Here's how the part is built. I have some questions about the finished solid (model axes, mm). Round coordinates to 2 decimals unless told otherwise and drop trailing zeros. Write each loop counter-clockwise with the first axis right and the second up, starting at its lowest first coordinate (ties: lowest second). Pieces come first, ordered by that corner, then holes. Notation, with made-up numbers: M 87,52.25 L 95,52.25 A27 ccw 95,80.25 Z; hole C 54,1.5 d4. An arc over 180 degrees is marked long. Use a Markdown table: item, result. Add a question column.
```python
from build123d import *

# Parameters (mm, degrees)
F0_R        = 7.2334484139
F1_DEPTH    = 67.7
F2_R        = 15.3458789883
F3_DEPTH    = 21.4
F4_R        = 2
F5_S5_R     = 7.2334484139
F5_T6_DEPTH = 24
F6_R        = 5


# Not quite as in the source:
# - a fillet or chamfer that OpenCascade refuses, or shapes differently, is made with other operations: its cross-section is extruded or revolved along the edge and cut away or added


with BuildPart() as f1:
    # F0 (on Top) → F1 (new body)
    with BuildSketch(Plane.XY):
        Circle(F0_R)
    extrude(amount=F1_DEPTH)

    # F2 (on Top) → F3 (join)
    with BuildSketch(Plane.XY):
        Circle(F2_R)
    extrude(amount=F3_DEPTH)

    # F4
    f4_edges = [f1.edges().sort_by_distance(p)[0] for p in [
        (-7.233448, 0, 67.7),
    ]]
    fillet(f4_edges, radius=F4_R)

    # F5: chamfer of 10 on 1 edges, made by hand


with BuildPart() as f5_tool2:
    # F5_s3 → F5_t4 (revolve)
    with BuildSketch(Plane.XZ):
        Polygon((5.3458789883, 21.4), (15.3458789883, 11.4), (15.3458789883, 21.4), align=None)
    revolve(axis=Axis((0, 0, 21.4), (0, 0, 1)))

    # F5_s5 → F5_t6 (cut, symmetric)
    with BuildSketch(Plane.XY.offset(16.4)):
        Circle(F5_S5_R)
    extrude(amount=F5_T6_DEPTH, both=True, mode=Mode.SUBTRACT)


with BuildPart() as f1_1:
    add(f1.part)

    # F5_t1: cut F5_tool2
    add(f5_tool2.part, mode=Mode.SUBTRACT)

    # F6
    f6_edges = [f1_1.edges().sort_by_distance(p)[0] for p in [
        (-15.345879, 0, 11.4),
    ]]
    fillet(f6_edges, radius=F6_R)


solid = f1_1.part
```
Item 1: I need wall thicknesses on probe 1 along Y at (x, z) = (-5, 44); probe 2 along X at (y, z) = (-4.5, 32.5); probe 3 along X at (y, z) = (-1.5, 6). Which ranges of each line are inside material? Lowest first, please. Write a range as from..to.
Item 2: Imagine slicing it at A-A on z = 34.5. List the corners of the cut face in (x, y) for me, plus the area to 3 significant figures.
Item 3: For pin 1 Ø8 at (y, z) = (10.5, 48.5) entering from -X; pin 2 Ø12 at (x, z) = (1.5, 17.5) entering from +Y; pin 3 Ø5 at (y, z) = (-12, 31.5) entering from +X; pin 4 Ø5 at (x, z) = (-9, 42.5) entering from +Y, each with a flat end and sliding along its axis, tell me the tip position at first contact or that it passes through.
The answers:
| question | item | result |
|---|---|---|
| 1 | probe 1 | -5.23..5.23 |
| 1 | probe 2 | -5.66..5.66 |
| 1 | probe 3 | -15.27..15.27 |
| 2 | outline | C 0,0 d14.47 |
| 2 | area | 164 mm² |
| 3 | pin 1 | x = -3.17 |
| 3 | pin 2 | y = 14.81 |
| 3 | pin 3 | through |
| 3 | pin 4 | y = 3.17 |
